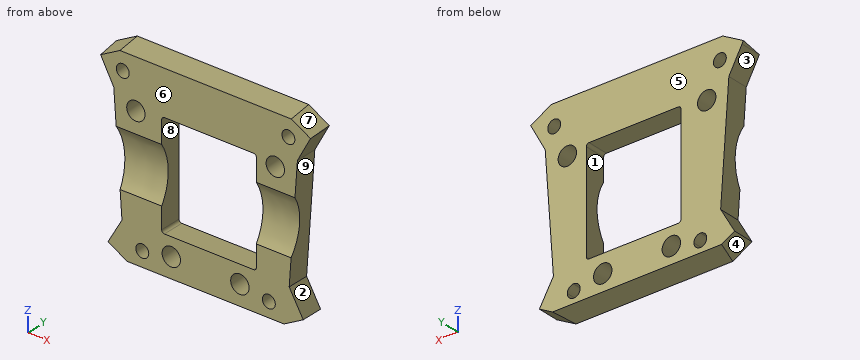
from build123d import *

# Parameters (mm, degrees)
BOSS_EXTRUDE1_DEPTH      = 10
CUT_EXTRUDE1_DEPTH       = 39.246851426
CUT_EXTRUDE1_DEPTH_BACK  = 39.246851426
BOSS_EXTRUDE2_DEPTH      = 31.226887
BOSS_EXTRUDE2_DEPTH_BACK = 31.226887
BOSS_EXTRUDE4_DEPTH      = 7.852901
CUT_EXTRUDE6_REACH       = 15.474
BOSS_EXTRUDE6_DEPTH      = 7.852901
CUT_EXTRUDE7_REACH       = 15.474
SKETCH15_W               = 34.5
SKETCH15_H               = 38
CUT_EXTRUDE8_DEPTH       = 8.852900758
FILLET1_R                = 1
SKETCH16_R               = 2.35
CUT_EXTRUDE9_DEPTH       = 7.852901
SKETCH18_R               = 3.35
CUT_EXTRUDE10_DEPTH      = 7.852901
CUT_EXTRUDE11_DEPTH      = 55.774002508
CUT_EXTRUDE11_DEPTH_BACK = 23.774002507


with BuildPart() as part:
    # Sketch1 → Boss-Extrude1 (new body)
    with BuildSketch(Plane(origin=(0, 0, 0), x_dir=(1, 0, 0), z_dir=(0, 1, 0))):
        Polygon((28.55688655, 32.59875814), (-28.55688655, 32.59875814), (-35.576851431, 28.714212738), (-30.467341853, 19.813019987), (-33.461967186, -22.544744449), (-38.246851426, -31.408872502), (-31.226886544, -35.293417903), (31.226886544, -35.293417903), (38.246851426, -31.408872502), (33.461967186, -22.544744449), (30.467341853, 19.813019987), (35.576851431, 28.714212738), align=None)
    extrude(amount=BOSS_EXTRUDE1_DEPTH)

    # Sketch3 → Cut-Extrude1 (cut, two sides)
    with BuildSketch(Plane(origin=(0, 0, 0), x_dir=(0, 0, -1), z_dir=(1, 0, 0))) as cut_extrude1_sk:
        Polygon((31.354413252, 7.852900712), (32.59875814, 0), (34.072271083, 0), (34.072271083, 12.681172501), (31.434287212, 12.681172501), (-35.293417903, 12.681172501), (-35.293417903, 10), (-35.293417903, 7.852900712), align=None)
    extrude(amount=CUT_EXTRUDE1_DEPTH, mode=Mode.SUBTRACT)
    extrude(cut_extrude1_sk.sketch, amount=-CUT_EXTRUDE1_DEPTH_BACK, mode=Mode.SUBTRACT)

    # Sketch5 → Boss-Extrude2 (add, two sides)
    with BuildSketch(Plane(origin=(0, 0, 0), x_dir=(0, 0, -1), z_dir=(1, 0, 0))) as boss_extrude2_sk:
        Polygon((-35.29341791, 0), (-35.293417904, 7.852900712), (-36.537762798, 7.852900712), align=None)
    extrude(amount=BOSS_EXTRUDE2_DEPTH)
    extrude(boss_extrude2_sk.sketch, amount=-BOSS_EXTRUDE2_DEPTH_BACK)

    # Sketch7 → Boss-Extrude4 (add)
    with BuildSketch(Plane(origin=(0, 7.852900712, 0), x_dir=(1, 0, 0), z_dir=(0, 1, 0))):
        Polygon((31.226886544, -35.293417903), (38.246851426, -31.408872502), (38.774002508, -32.361514754), (31.226886544, -36.537762798), align=None)
    extrude(amount=-BOSS_EXTRUDE4_DEPTH)

    # Cut-Extrude6: up to this face of the body (flat: up to its plane)
    cut_extrude6_end = Plane(part.part.faces().sort_by_distance((0.070807589, 7.852900712, 3.202963046))[0])
    # Sketch12 → Cut-Extrude6 (cut, up to the picked face)
    with BuildSketch(Plane(origin=(0, 0, 0), x_dir=(1, 0, 0), z_dir=(0, 0.987677308, 0.156504106)), mode=Mode.PRIVATE) as cut_extrude6_sk1:
        Polygon((30.896216351, -36.268243015), (31.226886544, -36.087519199), (38.774002508, -31.962733774), (39.457900831, -31.588957374), (38.940691815, -30.642620529), (31.226886544, -34.85850799), (30.896216351, -34.85850799), align=None)
    cut_extrude6_tool1 = split(extrude(cut_extrude6_sk1.sketch, amount=CUT_EXTRUDE6_REACH, mode=Mode.PRIVATE), bisect_by=cut_extrude6_end, keep=Keep.BOTH, mode=Mode.PRIVATE)
    add(cut_extrude6_tool1.solids().sort_by_distance((35.037296, -5.226434, 32.983357))[0], mode=Mode.SUBTRACT)

    # Sketch13 → Boss-Extrude6 (add)
    with BuildSketch(Plane(origin=(0, 7.852900712, 0), x_dir=(1, 0, 0), z_dir=(0, 1, 0))):
        Polygon((-31.226886544, -35.293417904), (-31.226886544, -36.537762798), (-38.774002507, -32.361514753), (-38.246851426, -31.408872502), align=None)
    extrude(amount=-BOSS_EXTRUDE6_DEPTH)

    # Cut-Extrude7: up to this face of the body (flat: up to its plane)
    cut_extrude7_end = Plane(part.part.faces().sort_by_distance((0, 7.852900712, 3.265184411))[0])
    # Sketch14 → Cut-Extrude7 (cut, up to the picked face)
    with BuildSketch(Plane(origin=(0, 0, 0), x_dir=(1, 0, 0), z_dir=(0, 0.987677308, 0.156504106)), mode=Mode.PRIVATE) as cut_extrude7_sk1:
        Polygon((-38.774002507, -31.962733773), (-31.226886544, -36.087519199), (-31.226886544, -34.858507985), (-39.138580492, -30.534466847), (-40.986059535, -30.753760618), align=None)
    cut_extrude7_tool1 = split(extrude(cut_extrude7_sk1.sketch, amount=CUT_EXTRUDE7_REACH, mode=Mode.PRIVATE), bisect_by=cut_extrude7_end, keep=Keep.BOTH, mode=Mode.PRIVATE)
    add(cut_extrude7_tool1.solids().sort_by_distance((-35.660699, -5.175776, 32.663656))[0], mode=Mode.SUBTRACT)

    # Sketch15 → Cut-Extrude8 (cut, through all)
    with BuildSketch(Plane(origin=(0, 7.852900712, 0), x_dir=(1, 0, 0), z_dir=(0, 1, 0))):
        with Locations((1.25, -0.19872767)):
            Rectangle(SKETCH15_W, SKETCH15_H)
    extrude(amount=-CUT_EXTRUDE8_DEPTH, mode=Mode.SUBTRACT)

    # Fillet1
    fillet1_edges = [part.edges().sort_by_distance(p)[0] for p in [
        (-16, 3.926450356, 19.19872767),
        (-16, 3.926450356, -18.80127233),
        (18.5, 3.926450356, -18.80127233),
        (18.5, 3.926450356, 19.19872767),
    ]]
    fillet(fillet1_edges, radius=FILLET1_R)

    # Sketch16 → Cut-Extrude9 (cut)
    with BuildSketch(Plane(origin=(0, 7.852900712, 0), x_dir=(1, 0, 0), z_dir=(0, 1, 0))):
        with BuildLine():
            ThreePointArc((-23.169283502, 24.901447562), (-23.167136672, 24.901345749), (-23.16498975, 24.901245899))
            ThreePointArc((-23.16498975, 24.901245899), (-21.433855825, 25.549266666), (-20.706886553, 27.248758135))
            ThreePointArc((-20.706886553, 27.248758135), (-24.678362296, 28.949733272), (-23.169283502, 24.901447563))
        make_face()
        with Locations((-30.183959547, -29.01317237)):
            Circle(SKETCH16_R)
        with Locations((30.183959554, -29.013172365)):
            Circle(SKETCH16_R)
        with BuildLine():
            ThreePointArc((23.164989747, 24.901245903), (23.167136669, 24.901345753), (23.169283499, 24.901447567))
            ThreePointArc((23.169283499, 24.901447567), (24.757861687, 25.627282396), (25.40688655, 27.24875814))
            ThreePointArc((25.40688655, 27.24875814), (21.357395081, 28.871788867), (23.164989747, 24.901245903))
        make_face()
    extrude(amount=-CUT_EXTRUDE9_DEPTH, mode=Mode.SUBTRACT)

    # Sketch18 → Cut-Extrude10 (cut)
    with BuildSketch(Plane(origin=(0, 7.852900712, 0), x_dir=(1, 0, 0), z_dir=(0, 1, 0))):
        with Locations((-25.397590164, -17.646835853)):
            Circle(SKETCH18_R)
        with Locations((12.500295063, 25.355028006)):
            Circle(SKETCH18_R)
        with Locations((-12.499704907, 25.353798513)):
            Circle(SKETCH18_R)
        with Locations((25.402409775, -17.644337524)):
            Circle(SKETCH18_R)
    extrude(amount=-CUT_EXTRUDE10_DEPTH, mode=Mode.SUBTRACT)

    # Sketch19 → Cut-Extrude11 (cut, two sides)
    with BuildSketch(Plane(origin=(-16, 0, 0), x_dir=(0, 0, -1), z_dir=(1, 0, 0))) as cut_extrude11_sk:
        with BuildLine():
            Line((-10.0632786, 0), (10.065144671, 0))
            add(Edge.make_bspline(
                [(0.000933035, 2.967511147), (0.544521725, 2.967511147), (1.619583471, 2.921196479), (3.854022546, 2.625629399), (6.684377205, 1.845878396), (8.927393688, 0.727415261), (10.014615597, 0.032640048), (10.065144671, 0)],
                knots=[0, 0, 0, 0, 0.0625, 0.125, 0.25, 0.375, 0.381109812, 0.381109812, 0.381109812, 0.381109812], degree=3))
            add(Edge.make_bspline(
                [(0.000933035, 2.967511147), (-0.542655654, 2.967511147), (-1.6177174, 2.921196479), (-3.852156475, 2.625629399), (-6.682511135, 1.845878396), (-8.925527618, 0.727415261), (-10.012749527, 0.032640048), (-10.0632786, 0)],
                knots=[0, 0, 0, 0, 0.0625, 0.125, 0.25, 0.375, 0.381109812, 0.381109812, 0.381109812, 0.381109812], degree=3))
        make_face()
    extrude(amount=CUT_EXTRUDE11_DEPTH, mode=Mode.SUBTRACT)
    extrude(cut_extrude11_sk.sketch, amount=-CUT_EXTRUDE11_DEPTH_BACK, mode=Mode.SUBTRACT)


solid = part.part
Can you work these out from the model? Positions are in its coordinate system, mm. Face numbers are marked on the shaded views. A direction names the side the tool comes from. Coordinates: 2 decimals unless noted, no trailing zeros. Write each loop counter-clockwise with the first axis right and the second up, starting at its lowest first coordinate (ties: lowest second). Pieces come first, ordered by that corner, then holes. Notation, with made-up numbers: (74.5, -1.5) -> (89.5, -1.5) arc R12 cw to (89.5, 10.5) -> close; hole circle Ø9 at (40, 29.25). An arc over 180 degrees is marked (long way). Write each question's results on one line, items separated by ' | '. Start each with the question number.
Q1. Imagine slicing it at C-C (z = 12.5). Write out the boundary of the cut face in (x, y), then the cut area to 3 significant figures.
Q2. Imagine slicing it at D-D (x = 12). Write out the boundary of the cut face in (y, z), then the cut area to 3 significant figures.
Q3. Imagine slicing it at A-A (x = -4.5). Write out the boundary of the cut face in (y, z).
Q4. We'd pull the mould along Z, two halves only. Please class the marked faces 6, 7, 8 and 9: +Z half, -Z half, draft (parallel to the pull), parting line (faces both ways), or undercut.
Q5. On a 3-axis mill with a long thin cutter (end or side, diameter ignored), from which of +Z, -Z, +X, -X, +Y, -Y can I reach the whole of each face in a straight line? I mean the marked faces 1, 2, 3, 4 and 5. Say none if no direction works.
Q6. If I drill on probe 1 along X at (y, z) = (0.5, 31); probe 2 along X at (y, z) = (6.5, -9); probe 3 along X at (y, z) = (6.5, 17), over which ranges is the centre line in solid material (lowest first)?
Q7. I'm going to push flat-ended pins straight in: pin 1 (1.5 mm diameter, centred on x = -18, y = 1.5, fed in from +Z); pin 2 (4 mm diameter, centred on x = 9, y = 2.5, fed in from -Z); pin 3 (2.5 mm diameter, centred on x = -3.5, y = 5.5, fed in from +Z). Where does each tip first touch, or does it pass through?
Q8. Imagine slicing it at B-B (y = 4). State how many separate pieces and enclosed holes the cut face has, then the cut area to 3 significant figures.
Taken from the geometry:
1) outline: (-32.75, 0) -> (-16, 0) -> (-16, 7.85) -> (-32.75, 7.85) -> close; (18.5, 0) -> (32.75, 0) -> (32.75, 7.85) -> (18.5, 7.85) -> close | area: 243 mm^2
2) outline: (0, -32.6) -> (7.85, -31.35) -> (7.85, -28.67) -> (0, -28.67) -> close; (0, -22.04) -> (7.85, -22.04) -> (7.85, -18.8) -> (0, -18.8) -> close; (0, 19.2) -> (7.85, 19.2) -> (7.85, 36.54) -> (0, 35.29) -> close | area: 183 mm^2
3) outline: (0, -32.6) -> (7.85, -31.35) -> (7.85, -18.8) -> (0, -18.8) -> close; (0, 19.2) -> (7.85, 19.2) -> (7.85, 36.54) -> (0, 35.29) -> close
4) face 6: draft | face 7: +Z half | face 8: undercut | face 9: undercut
5) face 1: +Y, -Y | face 2: +X, +Y, -Y | face 3: -X, +Y, -Y | face 4: -Z, -X, +Y, -Y | face 5: +Z, -Z, +X, -X, +Y
6) probe 1: x = -38.03 to -31.44, -28.93 to 28.93, 31.44 to 38.03 | probe 2: x = -31.23 to -16, 18.5 to 31.23 | probe 3: x = -33.07 to -28.68, -22.11 to -16, 18.5 to 22.11, 28.69 to 33.07
7) pin 1: stops at z = 35.65 | pin 2: stops at z = -32.52 | pin 3: stops at z = 36.36
8) separate pieces: 1 | enclosed holes: 9 | area: 2,940 mm^2
